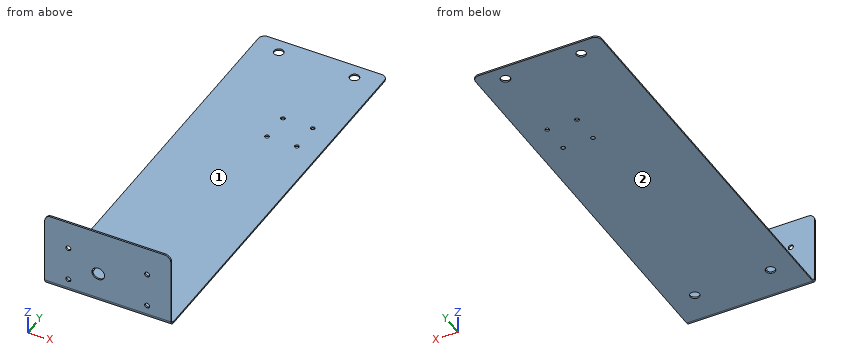
```python
from build123d import *

# Parameters (mm, degrees)
SKETCH2_W            = 127
SKETCH2_H            = 406.4
BOSS_EXTRUDE1_DEPTH  = 3.175
SKETCH3_W            = 127
SKETCH3_H            = 3.175
BOSS_EXTRUDE2_DEPTH  = 76.2
FILLET1_R            = 3.175
FILLET2_R            = 6.35
SKETCH4_R            = 6.35
SKETCH4_R_2          = 2.54
CUT_EXTRUDE1_DEPTH   = 416.840163104
SKETCH5_R            = 2.15
SKETCH5_R_2          = 4.7625
CUT_EXTRUDE2_DEPTH   = 227.117071448
CONVERT_SOLID1_START = -63.5
CONVERT_SOLID1_DEPTH = 127


# Read off the part's stored shape, not the designer's step: Convert-Solid1
with BuildPart() as part:
    # Sketch2 → Boss-Extrude1 (new body)
    with BuildSketch(Plane.XY):
        Rectangle(SKETCH2_W, SKETCH2_H)
    extrude(amount=BOSS_EXTRUDE1_DEPTH)

    # Sketch3 → Boss-Extrude2 (add)
    with BuildSketch(Plane.XY.offset(3.175)):
        with Locations((0, -201.6125)):
            Rectangle(SKETCH3_W, SKETCH3_H)
    extrude(amount=BOSS_EXTRUDE2_DEPTH)

    # Fillet1
    fillet1_edges = [part.edges().sort_by_distance(p)[0] for p in [
        (0, -200.025, 3.175),
        (0, -203.2, 0),
    ]]
    fillet(fillet1_edges, radius=FILLET1_R)

    # Fillet2
    fillet2_edges = [part.edges().sort_by_distance(p)[0] for p in [
        (-63.5, -201.6125, 79.375),
        (63.5, -201.6125, 79.375),
        (-63.5, 203.2, 1.5875),
        (63.5, 203.2, 1.5875),
    ]]
    fillet(fillet2_edges, radius=FILLET2_R)

    # Sketch4 → Cut-Extrude1 (cut, through all)
    with BuildSketch(Plane(origin=(0, -200.025, 0), x_dir=(1, 0, 0), z_dir=(0, 1, 0))):
        with Locations(Location((-9.525, -33.175, 0), (0, 0, 270))):
            Circle(SKETCH4_R)
        with Locations(Location((-39.6875, -15.7125, 0), (0, 0, 270))):
            Circle(SKETCH4_R_2)
        with Locations(Location((-39.6875, -50.6375, 0), (0, 0, 270))):
            Circle(SKETCH4_R_2)
        with Locations(Location((39.6875, -15.7125, 0), (0, 0, 270))):
            Circle(SKETCH4_R_2)
        with Locations(Location((39.6875, -50.6375, 0), (0, 0, 270))):
            Circle(SKETCH4_R_2)
    extrude(amount=-CUT_EXTRUDE1_DEPTH, mode=Mode.SUBTRACT)

    # Sketch5 → Cut-Extrude2 (cut, through all)
    with BuildSketch(Plane.XY.offset(3.175)):
        with Locations((10.273, 76.475)):
            Circle(SKETCH5_R)
        with Locations((40.273, 76.475)):
            Circle(SKETCH5_R)
        with Locations((40.273, 106.175)):
            Circle(SKETCH5_R)
        with Locations((10.273, 106.175)):
            Circle(SKETCH5_R)
        with Locations((-38.1, 187.96)):
            Circle(SKETCH5_R_2)
        with Locations((38.1, 187.96)):
            Circle(SKETCH5_R_2)
        with Locations((-38.1, -165.1)):
            Circle(SKETCH5_R_2)
        with Locations((38.1, -165.1)):
            Circle(SKETCH5_R_2)
    extrude(amount=-CUT_EXTRUDE2_DEPTH, mode=Mode.SUBTRACT)

    # Convert-Solid1 outline → Convert-Solid1 (cut)
    with BuildSketch(Plane.YZ.offset(CONVERT_SOLID1_START)):
        with BuildLine():
            ThreePointArc((-196.85, 1.5875), (-200.217596045, 2.982403955), (-201.6125, 6.35))
            Line((-201.6125, 6.35), (-201.6125, 79.375))
            Line((-201.6125, 79.375), (-203.2, 79.375))
            Line((-203.2, 79.375), (-203.2, 3.175))
            ThreePointArc((-203.2, 3.175), (-202.27006403, 0.92993597), (-200.025, 0))
            Line((-200.025, 0), (203.2, 0))
            Line((203.2, 0), (203.2, 1.5875))
            Line((203.2, 1.5875), (-196.85, 1.5875))
        make_face()
    extrude(amount=CONVERT_SOLID1_DEPTH, mode=Mode.SUBTRACT)


solid = part.part
```
Read the model definition and answer for the solid it produces. Units are mm, in the model's axes. Face numbers are marked on the shaded views. A direction names the side the tool comes from. Give positions to 0.01 mm unless a question says otherwise; leave off trailing zeros. Order: outer loops, then holes, each group sorted by start corner. A loop starts at its lowest first (then second) coordinate and runs counter-clockwise, first axis right, second up.
(1) Find section A-A (y = 187.96). Give the vertices of the cut face in (x, z) (1 decimal).
(2) For the marked faces 1 and 2, determine the directions among +Z, -Z, +X, -X, +Y, -Y from which every point of the face is accessible in a straight line to the end or side of a thin tool.
(3) Find section C-C (z = 57.5). Give the vertices of the cut face in (x, y) (1 decimal), plus the area to 3 significant figures.
(4) Find section D-D (y = 20). Give the vertices of the cut face in (x, z) (1 decimal).
(5) Straight lines are drawn through the part: L1, parallel to Z at x = -27.5, y = -137 (1 decimal); L2, parallel to Y at x = 8, z = 17.5 (1 decimal). For each, find the intervals that lie inside material, in ascending order.
(6) Given pin 1 (16.5 mm diameter, centred on x = -9.525, z = 33.175, fed in from +Y) (3 decimals); pin 2 (1 mm diameter, centred on x = 15.5, y = 125.5, fed in from +Z) (3 decimals), each flat-ended and moving along its own axis, determine where each tip first touches the part or whether it passes through.
Result sheet:
1. outline: (-63.5, 1.6) - (-42.9, 1.6) - (-42.9, 3.2) - (-63.5, 3.2) - close; (-33.3, 1.6) - (33.3, 1.6) - (33.3, 3.2) - (-33.3, 3.2) - close; (42.9, 1.6) - (63.5, 1.6) - (63.5, 3.2) - (42.9, 3.2) - close
2. face 1: +Z, +X, -X, +Y
2. face 2: -Z, +X, -X, +Y, -Y
3. outline: (-63.5, -201.6) - (63.5, -201.6) - (63.5, -200) - (-63.5, -200) - close
3. area: 202 mm2
4. outline: (-63.5, 1.6) - (63.5, 1.6) - (63.5, 3.2) - (-63.5, 3.2) - close
5. L1: z = 1.6 to 3.2
5. L2: y = -201.6 to -200
6. pin 1: stops at y = -200.025
6. pin 2: stops at z = 3.175
